```python
from build123d import *

# Parameters (mm, degrees)
F3_D = 50.8
F4_R = 10.16


with BuildPart() as f1:
    # F0 (on Front) → F1 (revolve)
    with BuildSketch(Plane.XZ):
        Polygon((-58.9493140578, 25.4), (-58.9493140578, -50.8), (68.0506859422, -50.8), (68.0506859422, 0), (4.5506859422, 0), (4.5506859422, 25.4), align=None)
    revolve(axis=Axis((-58.9493140578, 0, -12.7), (0, 0, -1)))

    # F3 (through all)
    with Locations(Plane.XY.offset(25.4)):
        with Locations((-58.9493140578, 0)):
            Hole(F3_D / 2)

    # F4
    f4_edges = [f1.edges().sort_by_distance(p)[0] for p in [
        (-185.949314, 0, 0),
    ]]
    fillet(f4_edges, radius=F4_R)


solid = f1.part
```
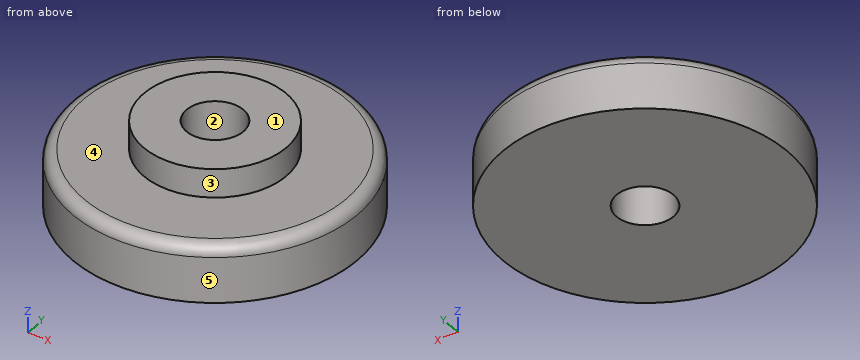
Verification items for the finished model (mm, model axes). Face numbers are marked on the shaded views. A direction names the side the tool comes from. Round coordinates to 2 decimals unless told otherwise and drop trailing zeros. Write each loop counter-clockwise with the first axis right and the second up, starting at its lowest first coordinate (ties: lowest second). Pieces come first, ordered by that corner, then holes.
1. Scan lines: L1, parallel to Y at x = -79.5, z = -43.5; L2, parallel to Z at x = 12.5, y = -92; L3, parallel to X at y = 110, z = -29. Record each from-to range of solid material in increasing order.
2. Section check A-A on y = 0. Enter the section's corners in (x, z).
3. Section check C-C on z = -24.5. Enter the section's corners in (x, y), plus the area to 3 significant figures.
4. Section check B-B on z = -6. Enter the section's corners in (x, y), plus the area to 3 significant figures.
5. Draft check along X on the marked faces 1, 2 and 3. Enter one of: +X half, -X half, draft (parallel to the pull), parting line (faces both ways), or undercut.
6. Access from +Z, -Z, +X, -X, +Y, -Y to the whole of each face (thin tool, end or side, straight path). Record for the marked faces 4 and 5.
7. Gauge pin test, flat ends, axial feed: P1, Ø5, axis at y = 30, z = -39, coming from the -X side; P2, Ø10, axis at x = -2, y = 30, coming from the +Z side; P3, Ø1.5, axis at y = 82.5, z = -19, coming from the -X side; P4, Ø6, axis at x = 2.5, z = -15.5, coming from the -Y side. Record the tip position at first contact, or that the pin passes through.
Answer:
1. L1: y = -125.33 to -14.93, 14.93 to 125.33
1. L2: z = -50.8 to 0
1. L3: x = -122.42 to 4.53
2. outline: (-185.95, -50.8) - (-84.35, -50.8) - (-84.35, 25.4) - (-122.45, 25.4) - (-122.45, 0) - (-175.79, 0) arc R10.16 ccw to (-185.95, -10.16) - close; (-33.55, -50.8) - (68.05, -50.8) - (68.05, -10.16) arc R10.16 ccw to (57.89, 0) - (4.55, 0) - (4.55, 25.4) - (-33.55, 25.4) - close
3. outline: circle Ø254 at (-58.95, 0); hole circle Ø50.8 at (-58.95, 0)
3. area: 48,600 mm2
4. outline: circle Ø252.22 at (-58.95, 0); hole circle Ø50.8 at (-58.95, 0)
4. area: 47,900 mm2
5. face 1: draft
5. face 2: undercut
5. face 3: parting line
6. face 4: +Z
6. face 5: +Z, -Z
7. P1: stops at x = -182.94
7. P2: stops at z = 25.4
7. P3: stops at x = -156.14
7. P4: stops at y = -112.75
